Read the model definition and answer for the solid it produces. Units are mm, in the model's axes. Face numbers are marked on the shaded views. Round coordinates to 2 decimals unless told otherwise and drop trailing zeros. Order: outer loops, then holes, each group sorted by start corner. A loop starts at its lowest first (then second) coordinate and runs counter-clockwise, first axis right, second up. Notation, with made-up numbers: (31, -11) -> (69, -11) arc R27 cw to (69, 6) -> close; hole circle Ø8 at (80.5, 53). An arc over 180 degrees is marked (long way). One line per item, written item: value. Start each with the question number.
1. Section A-A (y = -40.5) is taken. Give the vertices of the cut face in (x, z).
2. Flat-ended cylindrical pins translate along their axes: pin 1 Ø0.6 at (x, z) = (-53, 7) entering from -Y; pin 2 Ø1.1 at (x, y) = (-22.5, -33.5) entering from +Z; pin 3 Ø2.5 at (x, y) = (-58.5, 50) entering from +Z; pin 4 Ø3.5 at (y, z) = (-6, 7.5) entering from +X. Find the tip coordinate at first contact, or state that the pin passes through.
3. Section B-B (y = 22.5) is taken. Give the vertices of the cut face in (x, z), then the cut area to 3 significant figures.
4. Consider line 1 (Y direction, x = 22.5, z = 5.6); line 2 (Y direction, x = 38.5, z = 1.25); line 3 (X direction, y = 45.5, z = 10). Determine where each line is inside the solid, lowest interval first.
5. Section C-C (x = 1.5) is taken. Give the vertices of the cut face in (y, z), then the cut area to 3 significant figures.
6. The mould has two halves that part along X. Classify the marked faces 1 and 2: released by +X, released by -X, zero draft, split by the parting line, or undercut.
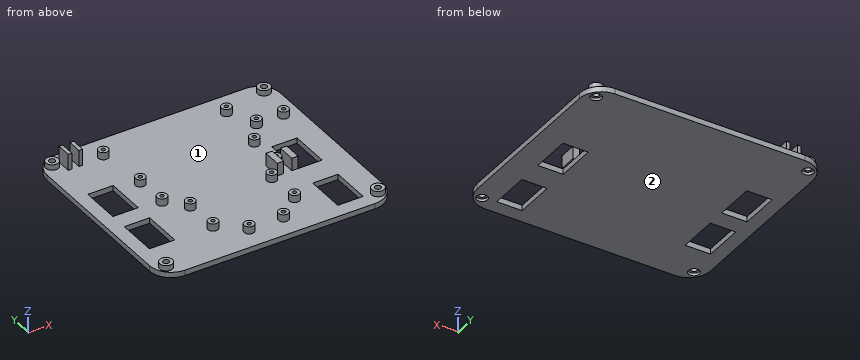
Autodesk Fusion 360 part; units mm, degrees
sketch "Sketch1" plane through (0, 0, 0) normal (0, 0, 1) x (1, 0, 0)
  line L0 (64.5, 57) -> (-64.5, 57)
  line L1 (-64.5, 57) -> (-64.5, -57)
  line L2 (-64.5, -57) -> (64.5, -57)
  line L3 (64.5, -57) -> (64.5, 57)
extrude "Extrude1" add sketch "Sketch1" along normal blind 3
fillet "Fillet1" radius 12 4 edges at (64.5, -57, 1.5) (-64.5, -57, 1.5) (-64.5, 57, 1.5) (64.5, 57, 1.5)
sketch "Sketch2" plane through (0, 0, 0) normal (0, 0, 1) x (1, 0, 0)
  line L0 (-43, 21) -> (-57, 21)
  line L1 (-57, 21) -> (-57, -1)
  line L2 (-57, -1) -> (-43, -1)
  line L3 (-43, -1) -> (-43, 21)
extrude "Extrude2" cut sketch "Sketch2" along normal blind 5 from surface at -1
sketch "Sketch3" plane through (0, 0, 0) normal (0, 0, 1) x (1, 0, 0)
  line L0 (-43, -11) -> (-57, -11)
  line L1 (-57, -11) -> (-57, -33)
  line L2 (-57, -33) -> (-43, -33)
  line L3 (-43, -33) -> (-43, -11)
extrude "Extrude3" cut sketch "Sketch3" along normal blind 5 from surface at -1
sketch "Sketch4" plane through (0, 0, 0) normal (0, 0, 1) x (1, 0, 0)
  line L0 (51, -27) -> (37, -27)
  line L1 (37, -27) -> (37, -49)
  line L2 (37, -49) -> (51, -49)
  line L3 (51, -49) -> (51, -27)
extrude "Extrude4" cut sketch "Sketch4" along normal blind 5 from surface at -1
sketch "Sketch5" plane through (0, 0, 0) normal (0, 0, 1) x (1, 0, 0)
  line L0 (51, 9) -> (37, 9)
  line L1 (37, 9) -> (37, -13)
  line L2 (37, -13) -> (51, -13)
  line L3 (51, -13) -> (51, 9)
extrude "Extrude5" cut sketch "Sketch5" along normal blind 5 from surface at -1
sketch "Sketch6" plane through (0, 0, 0) normal (0, 0, 1) x (1, 0, 0)
  circle A0 centre (-58.5, 50) radius 3.5
extrude "Extrude6" add sketch "Sketch6" along normal blind 3 from surface at 3
sketch "Sketch7" plane through (0, 0, 0) normal (0, 0, 1) x (1, 0, 0)
  circle A0 centre (-58.5, 50) radius 1.7
extrude "Extrude7" cut sketch "Sketch7" along normal blind 8 from surface at -1
sketch "Sketch8" plane through (0, 0, 0) normal (0, 0, 1) x (1, 0, 0)
  circle A0 centre (-58.5, 50) radius 3
extrude "Extrude8" cut sketch "Sketch8" along normal blind 1.5
sketch "Sketch9" plane through (0, 0, 0) normal (0, 0, 1) x (1, 0, 0)
  circle A0 centre (58.5, 50) radius 3.5
extrude "Extrude9" add sketch "Sketch9" along normal blind 3 from surface at 3
sketch "Sketch10" plane through (0, 0, 0) normal (0, 0, 1) x (1, 0, 0)
  circle A0 centre (58.5, 50) radius 1.7
extrude "Extrude10" cut sketch "Sketch10" along normal blind 8 from surface at -1
sketch "Sketch11" plane through (0, 0, 0) normal (0, 0, 1) x (1, 0, 0)
  circle A0 centre (58.5, 50) radius 3
extrude "Extrude11" cut sketch "Sketch11" along normal blind 1.5
sketch "Sketch12" plane through (0, 0, 0) normal (0, 0, 1) x (1, 0, 0)
  circle A0 centre (-58.5, -50) radius 3.5
extrude "Extrude12" add sketch "Sketch12" along normal blind 3 from surface at 3
sketch "Sketch13" plane through (0, 0, 0) normal (0, 0, 1) x (1, 0, 0)
  circle A0 centre (-58.5, -50) radius 1.7
extrude "Extrude13" cut sketch "Sketch13" along normal blind 8 from surface at -1
sketch "Sketch14" plane through (0, 0, 0) normal (0, 0, 1) x (1, 0, 0)
  circle A0 centre (-58.5, -50) radius 3
extrude "Extrude14" cut sketch "Sketch14" along normal blind 1.5
sketch "Sketch15" plane through (0, 0, 0) normal (0, 0, 1) x (1, 0, 0)
  circle A0 centre (58.5, -50) radius 3.5
extrude "Extrude15" add sketch "Sketch15" along normal blind 3 from surface at 3
sketch "Sketch16" plane through (0, 0, 0) normal (0, 0, 1) x (1, 0, 0)
  circle A0 centre (58.5, -50) radius 1.7
extrude "Extrude16" cut sketch "Sketch16" along normal blind 8 from surface at -1
sketch "Sketch17" plane through (0, 0, 0) normal (0, 0, 1) x (1, 0, 0)
  circle A0 centre (58.5, -50) radius 3
extrude "Extrude17" cut sketch "Sketch17" along normal blind 1.5
sketch "Sketch18" plane through (0, 0, 0) normal (0, 0, 1) x (1, 0, 0)
  circle A0 centre (-31.5, -3.5) radius 2.75
extrude "Extrude18" add sketch "Sketch18" along normal blind 4 from surface at 3
sketch "Sketch19" plane through (0, 0, 0) normal (0, 0, 1) x (1, 0, 0)
  circle A0 centre (-31.5, -3.5) radius 1.1
extrude "Extrude19" cut sketch "Sketch19" along normal blind 5 from surface at 3
sketch "Sketch20" plane through (0, 0, 0) normal (0, 0, 1) x (1, 0, 0)
  circle A0 centre (31.5, -3.5) radius 2.75
extrude "Extrude20" add sketch "Sketch20" along normal blind 4 from surface at 3
sketch "Sketch21" plane through (0, 0, 0) normal (0, 0, 1) x (1, 0, 0)
  circle A0 centre (31.5, -3.5) radius 1.1
extrude "Extrude21" cut sketch "Sketch21" along normal blind 5 from surface at 3
sketch "Sketch22" plane through (0, 0, 0) normal (0, 0, 1) x (1, 0, 0)
  circle A0 centre (-31.5, 15.5) radius 2.75
extrude "Extrude22" add sketch "Sketch22" along normal blind 4 from surface at 3
sketch "Sketch23" plane through (0, 0, 0) normal (0, 0, 1) x (1, 0, 0)
  circle A0 centre (-31.5, 15.5) radius 1.1
extrude "Extrude23" cut sketch "Sketch23" along normal blind 5 from surface at 3
sketch "Sketch24" plane through (0, 0, 0) normal (0, 0, 1) x (1, 0, 0)
  circle A0 centre (31.5, 15.5) radius 2.75
extrude "Extrude24" add sketch "Sketch24" along normal blind 4 from surface at 3
sketch "Sketch25" plane through (0, 0, 0) normal (0, 0, 1) x (1, 0, 0)
  circle A0 centre (31.5, 15.5) radius 1.1
extrude "Extrude25" cut sketch "Sketch25" along normal blind 5 from surface at 3
sketch "Sketch26" plane through (0, 0, 0) normal (0, 0, 1) x (1, 0, 0)
  circle A0 centre (-22.5, -34) radius 2.75
extrude "Extrude26" add sketch "Sketch26" along normal blind 4 from surface at 3
sketch "Sketch27" plane through (0, 0, 0) normal (0, 0, 1) x (1, 0, 0)
  circle A0 centre (-22.5, -34) radius 1.1
extrude "Extrude27" cut sketch "Sketch27" along normal blind 5 from surface at 3
sketch "Sketch28" plane through (0, 0, 0) normal (0, 0, 1) x (1, 0, 0)
  circle A0 centre (22.5, -34) radius 2.75
extrude "Extrude28" add sketch "Sketch28" along normal blind 4 from surface at 3
sketch "Sketch29" plane through (0, 0, 0) normal (0, 0, 1) x (1, 0, 0)
  circle A0 centre (22.5, -34) radius 1.1
extrude "Extrude29" cut sketch "Sketch29" along normal blind 5 from surface at 3
sketch "Sketch30" plane through (0, 0, 0) normal (0, 0, 1) x (1, 0, 0)
  circle A0 centre (-22.5, -14) radius 2.75
extrude "Extrude30" add sketch "Sketch30" along normal blind 4 from surface at 3
sketch "Sketch31" plane through (0, 0, 0) normal (0, 0, 1) x (1, 0, 0)
  circle A0 centre (-22.5, -14) radius 1.1
extrude "Extrude31" cut sketch "Sketch31" along normal blind 5 from surface at 3
sketch "Sketch32" plane through (0, 0, 0) normal (0, 0, 1) x (1, 0, 0)
  circle A0 centre (22.5, -14) radius 2.75
extrude "Extrude32" add sketch "Sketch32" along normal blind 4 from surface at 3
sketch "Sketch33" plane through (0, 0, 0) normal (0, 0, 1) x (1, 0, 0)
  circle A0 centre (22.5, -14) radius 1.1
extrude "Extrude33" cut sketch "Sketch33" along normal blind 5 from surface at 3
sketch "Sketch34" plane through (0, 0, 0) normal (0, 0, 1) x (1, 0, 0)
  circle A0 centre (-34, 44) radius 2.75
extrude "Extrude34" add sketch "Sketch34" along normal blind 4 from surface at 3
sketch "Sketch35" plane through (0, 0, 0) normal (0, 0, 1) x (1, 0, 0)
  circle A0 centre (-34, 44) radius 1.1
extrude "Extrude35" cut sketch "Sketch35" along normal blind 5 from surface at 3
sketch "Sketch36" plane through (0, 0, 0) normal (0, 0, 1) x (1, 0, 0)
  circle A0 centre (34, 44) radius 2.75
extrude "Extrude36" add sketch "Sketch36" along normal blind 4 from surface at 3
sketch "Sketch37" plane through (0, 0, 0) normal (0, 0, 1) x (1, 0, 0)
  circle A0 centre (34, 44) radius 1.1
extrude "Extrude37" cut sketch "Sketch37" along normal blind 5 from surface at 3
sketch "Sketch38" plane through (0, 0, 0) normal (0, 0, 1) x (1, 0, 0)
  circle A0 centre (-9.5, -45) radius 2.75
extrude "Extrude38" add sketch "Sketch38" along normal blind 4 from surface at 3
sketch "Sketch39" plane through (0, 0, 0) normal (0, 0, 1) x (1, 0, 0)
  circle A0 centre (-9.5, -45) radius 1.1
extrude "Extrude39" cut sketch "Sketch39" along normal blind 5 from surface at 3
sketch "Sketch40" plane through (0, 0, 0) normal (0, 0, 1) x (1, 0, 0)
  circle A0 centre (9.5, -45) radius 2.75
extrude "Extrude40" add sketch "Sketch40" along normal blind 4 from surface at 3
sketch "Sketch41" plane through (0, 0, 0) normal (0, 0, 1) x (1, 0, 0)
  circle A0 centre (9.5, -45) radius 1.1
extrude "Extrude41" cut sketch "Sketch41" along normal blind 5 from surface at 3
sketch "Sketch42" plane through (0, 0, 0) normal (0, 0, 1) x (1, 0, 0)
  circle A0 centre (40.5, 28) radius 2.75
extrude "Extrude42" add sketch "Sketch42" along normal blind 4 from surface at 3
sketch "Sketch43" plane through (0, 0, 0) normal (0, 0, 1) x (1, 0, 0)
  circle A0 centre (40.5, 28) radius 1.1
extrude "Extrude43" cut sketch "Sketch43" along normal blind 5 from surface at 3
sketch "Sketch44" plane through (0, 0, 0) normal (0, 0, 1) x (1, 0, 0)
  circle A0 centre (55.5, 28) radius 2.75
extrude "Extrude44" add sketch "Sketch44" along normal blind 4 from surface at 3
sketch "Sketch45" plane through (0, 0, 0) normal (0, 0, 1) x (1, 0, 0)
  circle A0 centre (55.5, 28) radius 1.1
extrude "Extrude45" cut sketch "Sketch45" along normal blind 5 from surface at 3
sketch "Sketch46" plane through (0, 0, 0) normal (0, 0, 1) x (1, 0, 0)
  line L0 (-52, 51) -> (-54, 51)
  line L1 (-54, 51) -> (-54, 43)
  line L2 (-54, 43) -> (-52, 43)
  line L3 (-52, 43) -> (-52, 51)
extrude "Extrude46" add sketch "Sketch46" along normal blind 9 from surface at 3
sketch "Sketch47" plane through (0, 0, 0) normal (0, 0, 1) x (1, 0, 0)
  line L0 (-46, 51) -> (-48, 51)
  line L1 (-48, 51) -> (-48, 43)
  line L2 (-48, 43) -> (-46, 43)
  line L3 (-46, 43) -> (-46, 51)
extrude "Extrude47" add sketch "Sketch47" along normal blind 9 from surface at 3
sketch "Sketch48" plane through (0, 0, 0) normal (0, 0, 1) x (1, 0, 0)
  line L0 (29.75, -3) -> (26.25, -3)
  line L1 (26.25, -3) -> (26.25, -13)
  line L2 (26.25, -13) -> (29.75, -13)
  line L3 (29.75, -13) -> (29.75, -3)
extrude "Extrude48" add sketch "Sketch48" along normal blind 7 from surface at 3
sketch "Sketch49" plane through (0, 0, 0) normal (0, 0, 1) x (1, 0, 0)
  line L0 (37.75, -3) -> (34.25, -3)
  line L1 (34.25, -3) -> (34.25, -13)
  line L2 (34.25, -13) -> (37.75, -13)
  line L3 (37.75, -13) -> (37.75, -3)
extrude "Extrude49" add sketch "Sketch49" along normal blind 7 from surface at 3
Answer:
1. outline: (-64.5, 0) -> (37, 0) -> (37, 3) -> (-64.5, 3) -> close; (51, 0) -> (64.5, 0) -> (64.5, 3) -> (51, 3) -> close
2. pin 1: y = 43
2. pin 2: z = 3
2. pin 3: through
2. pin 4: x = 37.75
3. outline: (-64.5, 0) -> (64.5, 0) -> (64.5, 3) -> (-64.5, 3) -> close
3. area: 387 mm^2
4. line 1: -36.75 to -35.1, -32.9 to -31.25, -16.75 to -15.1, -12.9 to -11.25
4. line 2: -57 to -49, -27 to -13, 9 to 57
4. line 3: -54 to -52, -48 to -46
5. outline: (-57, 0) -> (57, 0) -> (57, 3) -> (-57, 3) -> close
5. area: 342 mm^2
6. face 1: undercut
6. face 2: zero draft
